from build123d import *

# Parameters (mm, degrees)
EXTRUDE_1_DEPTH     = 1.6
SKETCH_2_R          = 3.5
SKETCH_2_R_2        = 2.5
EXTRUDE_2_DEPTH     = 2.6
SKETCH_7_R          = 1.5
CUT_EXTRUDE_1_DEPTH = 6


with BuildPart() as part:
    # 草图1 → 凸台-拉伸1 (new body)
    with BuildSketch(Plane.XY):
        with BuildLine():
            Line((-6.349999999, 7.050124355), (-3.5, 7.050124355))
            Line((-3.5, 7.050124355), (-1.936935669, 20.485344653))
            ThreePointArc((-1.936935669, 20.485344653), (0, 22.21), (1.936935669, 20.485344653))
            Line((1.936935669, 20.485344653), (3.5, 7.050124355))
            Line((3.5, 7.050124355), (6.349999999, 7.050124355))
            ThreePointArc((6.349999999, 7.050124355), (8.349999999, 5.050124355), (6.349999999, 3.050124355))
            Line((6.349999999, 3.050124355), (3.5, 3.050124355))
            Line((3.5, 3.050124355), (1.936935669, -10.385095943))
            ThreePointArc((1.936935669, -10.385095943), (0, -12.10975129), (-1.936935669, -10.385095943))
            Line((-1.936935669, -10.385095943), (-3.5, 3.050124355))
            Line((-3.5, 3.050124355), (-6.349999999, 3.050124355))
            ThreePointArc((-6.349999999, 3.050124355), (-8.349999999, 5.050124355), (-6.349999999, 7.050124355))
        make_face()
    extrude(amount=EXTRUDE_1_DEPTH)

    # 草图2 → 凸台-拉伸2 (add)
    with BuildSketch(Plane(origin=(0, 0, 0), x_dir=(-1, 0, 0), z_dir=(0, 0, -1))):
        with Locations((0, 5.05)):
            Circle(SKETCH_2_R)
        with Locations((0, 5.05)):
            Circle(SKETCH_2_R_2, mode=Mode.SUBTRACT)
    extrude(amount=EXTRUDE_2_DEPTH)

    # 草图7 → 切除-拉伸1 (cut)
    with BuildSketch(Plane(origin=(0, 0, 0), x_dir=(-1, 0, 0), z_dir=(0, 0, -1))):
        with Locations((0, 5.05)):
            Circle(SKETCH_7_R)
    extrude(amount=-CUT_EXTRUDE_1_DEPTH, mode=Mode.SUBTRACT)


solid = part.part
Can you work these out from the model? Positions are in its coordinate system, mm. A direction names the side the tool comes from. Coordinates: 2 decimals unless noted, no trailing zeros. Write each loop counter-clockwise with the first axis right and the second up, starting at its lowest first coordinate (ties: lowest second). Pieces come first, ordered by that corner, then holes.
Q1. Which directions (+Z, -Z, +X, -X, +Y, -Y) give clear straight access to the entire face, cutting with the end or side of a thin tool? Please do faces 1 (the face through (5, 7.05, 1)), 2 (the face through (-0.04, 22.21, 0.79)), 3 (the face through (5, 3.05, 1)), 4 (the face through (-8.35, 5.01, 0.79)), 5 (the face through (-1.34, 7.16, -1.28)).
Results found:
face 1: +Z, -Z, +X, +Y
face 2: +Z, -Z, +Y
face 3: +Z, -Z, +X, -Y
face 4: +Z, -Z, -X
face 5: -Z
Q2. Please list where these lines run through material, in increasing order: L1, parallel to Y at x = 0, z = 0.7; L2, parallel to Z at x = 0.25, y = -3; L3, parallel to Y at x = -6.5, z = 0.35.
Results found:
L1: y = -12.11 to 3.55, 6.55 to 22.21
L2: z = 0 to 1.6
L3: y = 3.06 to 7.04
Q3. For P1, Ø0.5, axis at x = -5, z = 0.5, coming from the -Y side; P2, Ø4, axis at x = 0, y = 5.05, coming from the -Z side; P3, Ø1.8, axis at x = -5.5, z = 0.5, coming from the +Y side, each with a flat end and sliding along its axis, tell me the tip position at first contact or that it passes through.
Results found:
P1: stops at y = 3.05
P2: stops at z = 0
P3: stops at y = 7.05
Q4. Imagine slicing it at B-B, the plane z = 1. List the corners of the cut face in (x, y) for me, plus the area to 3 significant figures.
Results found:
outline: (-6.35, 3.05) - (-3.5, 3.05) - (-1.94, -10.39) arc R1.95 ccw to (1.94, -10.39) - (3.5, 3.05) - (6.35, 3.05) arc R2 ccw to (6.35, 7.05) - (3.5, 7.05) - (1.94, 20.49) arc R1.95 ccw to (-1.94, 20.49) - (-3.5, 7.05) - (-6.35, 7.05) arc R2 ccw to start; hole circle Ø3 at (0, 5.05)
area: 213 mm2
Q5. Imagine slicing it at D-D, the plane y = 17.5. List the corners of the cut face in (x, z) for me, plus the area to 3 significant figures.
Results found:
outline: (-2.28, 0) - (2.28, 0) - (2.28, 1.6) - (-2.28, 1.6) - close
area: 7.31 mm2
Q6. Imagine slicing it at A-A, the plane x = 0. List the corners of the cut face in (y, z) for me, plus the area to 3 significant figures.
Results found:
outline: (-12.11, 0) - (1.55, 0) - (1.55, -2.6) - (2.55, -2.6) - (2.55, 0) - (3.55, 0) - (3.55, 1.6) - (-12.11, 1.6) - close; (6.55, 0) - (7.55, 0) - (7.55, -2.6) - (8.55, -2.6) - (8.55, 0) - (22.21, 0) - (22.21, 1.6) - (6.55, 1.6) - close
area: 55.3 mm2
Q7. If we mould it in two halves opening along X, with no side actions, what happens to faces 6 (the face through (-5, 7.05, 1)), 7 (the face through (-1.615, 1.945, -1.282)), 8 (the face through (0.195, 6.537, 0.789))? For each: +X half, -X half, draft (parallel to the pull), parting line (faces both ways), or undercut.
Results found:
face 6: draft
face 7: parting line
face 8: undercut
Q8. Imagine slicing it at C-C, the plane x = 5. List the corners of the cut face in (y, z) for me.
Results found:
outline: (3.05, 0) - (7.05, 0) - (7.05, 1.6) - (3.05, 1.6) - close
